Could you check a few things on this model? Use its own coordinates, in mm. A direction names the side the tool comes from. Coordinates: 2 decimals unless noted, no trailing zeros. Write each loop counter-clockwise with the first axis right and the second up, starting at its lowest first coordinate (ties: lowest second). Pieces come first, ordered by that corner, then holes. Notation, with made-up numbers: M 61.5,23.25 L 78.5,23.25 A33 ccw 78.5,56.25 Z; hole C -23.5,10 d5. An arc over 180 degrees is marked long. Answer as CSV lines item,"result". Start each with the question number.
Item 1: We'd pull the mould along X, two halves only. Please class faces 6 (the flat face through (-84, -19, -2.77)), 7 (the flat face through (-21, -28.13, -2)), 8 (the flat face through (-59.54, -15, -2)), 9 (the flat face through (71.627, -34, 1)): +X half, -X half, draft (parallel to the pull), parting line (faces both ways), or undercut.
Item 2: If I drill on line 1 along X through (y, z) = (-14, -1); line 2 along Y through (x, z) = (64.84, 0.95); line 3 along Y through (x, z) = (11.66, 1.05), over which ranges is the centre line in solid material (lowest first)? Write a range as [from, to].
Item 3: Suppose I cut it at C-C, the plane y = -50.59. Write out the boundary of the cut face in (x, z), and give its area (3 significant figures).
Item 4: Suppose I cut it at A-A, the plane x = 30.46. Write out the boundary of the cut face in (y, z), and give its area (3 significant figures).
Item 5: I'm going to push flat-ended pins straight in: P1, Ø0.8, axis at y = -9, z = -6.5, coming from the -X side; P2, Ø3.5, axis at x = -85, y = -25, coming from the -Z side; P3, Ø3.5, axis at y = -10.5, z = -5.5, coming from the +X side. Where does each tip first touch, or does it pass through?
Item 6: On a 3-axis mill with a long thin cutter (end or side, diameter ignored), from which of +Z, -Z, +X, -X, +Y, -Y can I reach the whole of each face in a straight line? I mean faces 1 (the flat face through (-84, -36.73, -1)), 2 (the flat face through (-10, -41, 3)), 3 (the flat face through (24.46, -16, -4)), 4 (the flat face through (-65.54, -16, -4)), 5 (the flat face through (18.46, -15, -2)). Say none if no direction works.
Item 7: Suppose I cut it at D-D, the plane x = -8. Write out the boundary of the cut face in (y, z).
Item 8: Suppose I cut it at B-B, the plane y = -14.73. Write out the boundary of the cut face in (x, z).
Autodesk Inventor part; units mm, degrees
ref_plane "Arbeitsebene2" through (-89.84, -42.13, -2.77) normal (0, 0, 1) x (1, 0, 0)
ref_plane "Arbeitsebene3" through (-58.54, -27.13, -6.3955) normal (0, 0, -1) x (0, 1, 0)
ref_plane "YZ Plane" through (0, 0, 0) normal (1, 0, 0) x (0, 1, 0)
ref_plane "Arbeitsebene1" through (0, 0, 0) normal (0, 0, 1) x (1, 0, 0)
sketch "Skizze1" plane through (0, 0, 0) normal (0, 0, 1) x (1, 0, 0)
  circle A0 centre (-54.34, -50.59) radius 1.5
  circle A1 centre (11.66, -50.59) radius 1.5
  circle A2 centre (-85.34, -22.83) radius 1
  circle A3 centre (-85.34, -22.83) radius 1 construction
  circle A4 centre (-85.34, 37.77) radius 1 construction
  line L0 (37.14, -42.13) -> (37.14, -36.73) construction
  arc A5 (32.14, -41.73) -> (37.14, -36.73) centre (32.14, -36.73) ccw construction
  line L1 (32.14, -41.73) -> (-73.22, -41.73) construction
  arc A6 (-78.22, -36.73) -> (-73.22, -41.73) centre (-73.22, -36.73) ccw construction
  line L2 (-78.22, -36.73) -> (-78.22, 48.27) construction
  arc A7 (-73.22, 53.27) -> (-78.22, 48.27) centre (-73.22, 48.27) ccw construction
  line L3 (-73.22, 53.27) -> (32.14, 53.27) construction
  arc A8 (37.14, 48.27) -> (32.14, 53.27) centre (32.14, 48.27) ccw construction
  line L4 (37.14, 48.27) -> (37.14, 54.21) construction
  line L5 (37.14, 54.21) -> (-89.84, 54.21) construction
  line L6 (-89.84, 54.21) -> (-89.84, -42.13) construction
  line L7 (-89.84, -42.13) -> (37.14, -42.13) construction
  circle A9 centre (64.84, -24.91) radius 1.5 construction
  circle A10 centre (-85.34, -43.41) radius 1 construction
  circle A11 centre (64.84, 35.59) radius 1.5 construction
  circle A12 centre (11.66, -50.59) radius 1.5 construction
  circle A13 centre (-54.34, -50.59) radius 1.5 construction
  circle A14 centre (-85.34, 58.59) radius 1 construction
  line L8 (-89.84, 67.09) -> (-89.84, 54.21) construction
  line L9 (-89.84, 54.21) -> (37.14, 54.21) construction
  line L10 (37.14, 54.21) -> (37.14, -42.13) construction
  line L11 (37.14, -42.13) -> (-89.84, -42.13) construction
  line L12 (-89.84, -42.13) -> (-89.84, -67.09) construction
  line L13 (-89.84, -67.09) -> (89.84, -67.09) construction
  line L14 (89.84, -67.09) -> (89.84, 67.09) construction
  line L15 (89.84, 67.09) -> (-89.84, 67.09) construction
  line L16 (-58.54, -1.33) -> (17.46, -1.33) construction
  line L17 (-58.54, -27.13) -> (-58.54, -1.33) construction
  line L18 (17.46, -27.13) -> (-58.54, -27.13) construction
  line L19 (17.46, -1.33) -> (17.46, -27.13) construction
  line L20 (-89.84, -1.33) -> (-59.54, -1.33)
  line L21 (-59.54, -1.33) -> (-59.54, -28.13)
  line L22 (-59.54, -28.13) -> (18.46, -28.13)
  line L23 (18.46, -28.13) -> (18.46, -1.33)
  line L24 (18.46, -1.33) -> (71.6268, -1.33)
  line L25 (71.6268, -1.33) -> (71.6268, -67.09)
  line L26 (71.6268, -67.09) -> (-89.84, -67.09)
  line L27 (-89.84, -1.33) -> (-89.84, -67.09)
  circle A15 centre (-54.34, -50.59) radius 1.5
  circle A16 centre (11.66, -50.59) radius 1.5
  circle A17 centre (-85.34, -22.83) radius 1
  circle A18 centre (64.84, -24.91) radius 1.5
  point P0 (0, 0)
  dimension "d0" = 1
  dimension "d1" = 1
  dimension "d2" = 1
extrude "Extrusion1" add sketch "Skizze1" along normal blind 3
sketch "Skizze2" plane through (0, 0, 0) normal (0, 0, -1) x (-1, 0, 0)
  circle A0 centre (85.34, -22.83) radius 1
  circle A1 centre (85.34, 37.77) radius 1
  line L0 (-37.14, -42.13) -> (-37.14, -36.73)
  arc A2 (-37.14, -36.73) -> (-32.14, -41.73) centre (-32.14, -36.73) ccw
  line L1 (-32.14, -41.73) -> (73.22, -41.73)
  arc A3 (73.22, -41.73) -> (78.22, -36.73) centre (73.22, -36.73) ccw
  line L2 (78.22, -36.73) -> (78.22, 48.27)
  arc A4 (78.22, 48.27) -> (73.22, 53.27) centre (73.22, 48.27) ccw
  line L3 (73.22, 53.27) -> (-32.14, 53.27)
  arc A5 (-32.14, 53.27) -> (-37.14, 48.27) centre (-32.14, 48.27) ccw
  line L4 (-37.14, 48.27) -> (-37.14, 54.21)
  line L5 (-37.14, 54.21) -> (89.84, 54.21)
  line L6 (89.84, 54.21) -> (89.84, -42.13)
  line L7 (89.84, -42.13) -> (-37.14, -42.13)
  line L8 (78.22, -36.73) -> (89.84, -36.73)
  line L9 (89.84, -1.33) -> (89.84, -67.09)
  line L10 (59.54, -1.33) -> (89.84, -1.33)
  line L11 (89.84, -36.73) -> (78.8105, -36.73)
  line L12 (78.8105, -36.73) -> (78.8105, -1.33)
  line L13 (78.8105, -1.33) -> (89.84, -1.33)
  line L14 (89.84, -1.33) -> (89.84, -36.73)
  point P0 (0, 0)
ref_plane "Arbeitsebene2" through (-89.84, -42.13, -2.77) normal (0, 0, 1) x (1, 0, 0)
extrude "Extrusion2" add sketch "Skizze2" along normal up to surface (2.77 mm away) contours L8 L12 L10 L6
ref_plane "Arbeitsebene3" through (-58.54, -27.13, -6.3955) normal (0, 0, -1) x (0, 1, 0)
sketch "Skizze3" plane through (0, 0, 0) normal (0, 0, -1) x (-1, 0, 0)
  line L0 (78.8105, -36.73) -> (78.8105, -1.33)
  line L1 (59.54, -1.33) -> (78.8105, -1.33)
  line L2 (59.54, -28.13) -> (59.54, -1.33)
  line L3 (-18.46, -28.13) -> (59.54, -28.13)
  line L4 (-18.46, -1.33) -> (-18.46, -28.13)
  line L5 (-71.6268, -1.33) -> (-18.46, -1.33)
  line L6 (-71.6268, -67.09) -> (-71.6268, -1.33)
  line L7 (89.84, -67.09) -> (-71.6268, -67.09)
  line L8 (89.84, -36.73) -> (89.84, -67.09)
  line L9 (89.84, -36.73) -> (78.8105, -36.73)
  circle A0 centre (-64.84, -24.91) radius 1.5
  circle A1 centre (-11.66, -50.59) radius 1.5
  circle A2 centre (54.34, -50.59) radius 1.5
  line L10 (-18.46, -1.33) -> (-18.46, -28.13)
  line L11 (-18.46, -1.33) -> (-24.46, -1.33)
  line L12 (-24.46, -1.33) -> (-24.46, -28.13)
  line L13 (-24.46, -28.13) -> (-18.46, -28.13)
  line L14 (-18.46, -28.13) -> (-18.46, -1.33)
  line L15 (59.54, -1.33) -> (65.54, -1.33)
  line L16 (65.54, -1.33) -> (65.54, -28.13)
  line L17 (65.54, -28.13) -> (59.54, -28.13)
  line L18 (59.54, -28.13) -> (59.54, -1.33)
  line L19 (65.54, -28.13) -> (-24.46, -28.13)
  line L20 (-24.46, -28.13) -> (-24.46, -30.13)
  line L21 (-24.46, -30.13) -> (65.54, -30.13)
  line L22 (65.54, -30.13) -> (65.54, -28.13)
  point P0 (0, 0)
  dimension "d7" = 6
  dimension "d8" = 6
  dimension "d9" = 2
extrude "Extrusion3" add sketch "Skizze3" along normal up to surface (6.3955 mm away) contours L16 L17 L2 L1 | L22 L21 L20 L13 L3 L17 | L13 L12 L5 L4
sketch "Skizze4" plane through (0, 0, -6.3955) normal (0, 0, -1) x (-1, 0, 0)
  line L0 (-18.46, -1.33) -> (-24.46, -1.33)
  line L1 (-24.46, -1.33) -> (-24.46, -30.13)
  line L2 (-24.46, -30.13) -> (65.54, -30.13)
  line L3 (65.54, -30.13) -> (65.54, -1.33)
  line L4 (65.54, -1.33) -> (59.54, -1.33)
  line L5 (59.54, -1.33) -> (59.54, -28.13)
  line L6 (59.54, -28.13) -> (-18.46, -28.13)
  line L7 (-18.46, -28.13) -> (-18.46, -1.33)
  line L8 (59.54, -1.33) -> (53.54, -1.33)
  line L9 (53.54, -1.33) -> (53.54, -28.13)
  line L10 (53.54, -28.13) -> (59.54, -28.13)
  line L11 (59.54, -28.13) -> (59.54, -1.33)
  line L12 (-18.46, -28.13) -> (59.54, -28.13)
  line L13 (-18.46, -28.13) -> (-12.46, -28.13)
  line L14 (-12.46, -28.13) -> (-12.46, -1.33)
  line L15 (-12.46, -1.33) -> (-18.46, -1.33)
  line L16 (-18.46, -1.33) -> (-18.46, -28.13)
  line L17 (-12.46, -28.13) -> (53.54, -28.13)
  line L18 (53.54, -28.13) -> (53.54, -26.13)
  line L19 (53.54, -26.13) -> (-12.46, -26.13)
  line L20 (-12.46, -26.13) -> (-12.46, -28.13)
  point P0 (0, 0)
  point P1 (-12.46, -26.13)
  dimension "d12" = 6
  dimension "d13" = 6
  dimension "d14" = 2
extrude "Extrusion4" add sketch "Skizze4" along normal blind 1
sketch "Skizze5" plane through (0, 0, 3) normal (0, 0, 1) x (1, 0, 0)
  line L0 (-89.84, -67.09) -> (71.6268, -67.09)
  line L1 (71.6268, -67.09) -> (71.6268, -1.33)
  line L2 (71.6268, -1.33) -> (18.46, -1.33)
  line L3 (18.46, -1.33) -> (18.46, -28.13)
  line L4 (18.46, -28.13) -> (-59.54, -28.13)
  line L5 (-59.54, -28.13) -> (-59.54, -1.33)
  line L6 (-59.54, -1.33) -> (-89.84, -1.33)
  line L7 (-89.84, -1.33) -> (-89.84, -67.09)
  circle A0 centre (64.84, -24.91) radius 1.5
  circle A1 centre (-85.34, -22.83) radius 1
  circle A2 centre (11.66, -50.59) radius 1.5
  circle A3 centre (-54.34, -50.59) radius 1.5
  circle A4 centre (-71.54, -14.73) radius 1.4
  circle A5 centre (30.46, -14.73) radius 1.4
  point P0 (0, 0)
  dimension "d18" = 2.8
  dimension "d19" = 2.8
  dimension "d20" = 12
  dimension "d21" = 12
extrude "Extrusion5" cut sketch "Skizze5" against normal through all contours A4 | A5
properties part number "30_XYTabel_Aliexpress_cellSTORM_chiptray"
Ans:
1,face 6,"draft"
1,face 7,"undercut"
1,face 8,"undercut"
1,face 9,"+X half"
2,line 1,"x = [-89.84, -78.81], [-65.54, -59.54], [18.46, 24.46]"
2,line 2,"y = [-67.09, -26.41], [-23.41, -1.33]"
2,line 3,"y = [-67.09, -52.09], [-49.09, -28.13]"
3,outline,"M -89.84,0 L -55.84,0 L -55.84,3 L -89.84,3 Z; M -52.84,0 L 10.16,0 L 10.16,3 L -52.84,3 Z; M 13.16,0 L 71.63,0 L 71.63,3 L 13.16,3 Z"
3,area,"466 mm^2"
4,outline,"M -67.09,0 L -16.13,0 L -16.13,3 L -67.09,3 Z; M -13.33,0 L -1.33,0 L -1.33,3 L -13.33,3 Z"
4,area,"189 mm^2"
5,P1,"stops at x = -65.54"
5,P2,"stops at z = -2.77"
5,P3,"stops at x = 24.46"
6,face 1,"-Z, +X, -X, -Y"
6,face 2,"+Z, +X, -X, +Y, -Y"
6,face 3,"-Z, +X, +Y, -Y"
6,face 4,"-Z, +Y, -Y"
6,face 5,"+Z, +Y"
7,outline,"M -67.09,0 L -30.13,0 L -30.13,-7.4 L -26.13,-7.4 L -26.13,-6.4 L -28.13,-6.4 L -28.13,3 L -67.09,3 Z"
8,outline,"M -89.84,-2.77 L -78.81,-2.77 L -78.81,0 L -72.94,0 L -72.94,3 L -89.84,3 Z; M -70.14,0 L -65.54,0 L -65.54,-7.4 L -53.54,-7.4 L -53.54,-6.4 L -59.54,-6.4 L -59.54,3 L -70.14,3 Z; M 12.46,-7.4 L 24.46,-7.4 L 24.46,0 L 29.06,0 L 29.06,3 L 18.46,3 L 18.46,-6.4 L 12.46,-6.4 Z; M 31.86,0 L 71.63,0 L 71.63,3 L 31.86,3 Z"
